from build123d import *

# Parameters (mm, degrees)
F0_W     = 105.55254668
F0_H     = 105.5525541306
F1_DEPTH = 99.314
F3_DEPTH = 104.14
F4_W     = 27.6781544089
F4_H     = 48.5944971442
F5_DEPTH = 3.81
F6_R     = 12.9022285529
F7_DEPTH = 4.826


with BuildPart() as f1:
    # F0 (on Top) → F1 (new body)
    with BuildSketch(Plane.XY):
        with Locations((0.8764155209, -6.7373067141)):
            Rectangle(F0_W, F0_H)
    extrude(amount=F1_DEPTH)

    # F2 (on face) → F3 (join)
    with BuildSketch(Plane(origin=(-51.8998578191, 0, 0), x_dir=(0, -1, 0), z_dir=(-1, 0, 0))):
        Polygon((12.3477084562, 113.1768599153), (-46.0389703512, 99.314), (59.5135837793, 99.314), align=None)
    extrude(amount=-F3_DEPTH)

    # F4 (on face) → F5 (cut)
    with BuildSketch(Plane.YZ.offset(53.6526888609)):
        with Locations((-5.462795496, 24.2972485721)):
            Rectangle(F4_W, F4_H)
    extrude(amount=-F5_DEPTH, mode=Mode.SUBTRACT)

    # F6 (on face) → F7 (cut)
    with BuildSketch(Plane.YZ.offset(53.6526888609)):
        with Locations((-9.2169223353, 78.1042650342)):
            Circle(F6_R)
    extrude(amount=-F7_DEPTH, mode=Mode.SUBTRACT)


solid = f1.part
For this review, take the finished solid that the model builds, in its own axes (mm). A direction names the side the tool comes from. Round coordinates to 2 decimals unless told otherwise and drop trailing zeros. Write each loop counter-clockwise with the first axis right and the second up, starting at its lowest first coordinate (ties: lowest second). Pieces come first, ordered by that corner, then holes. Notation, with made-up numbers: (41.25, -30) - (60.25, -30) arc R13 ccw to (60.25, -15) - close; hole circle Ø6 at (53, 64). An arc over 180 degrees is marked (long way). Write item = value, one per line. Start each with the question number.
1. Consider section D-D on z = 102.5. State the section outline as (x, y) points.
2. For faces 4 (the face through (48.827, -9, 78)), 5 (the face through (49.843, -6, 25)), 6 (the face through (52.24, -6, 103)), list the 3-axis set-ups (+Z, -Z, +X, -X, +Y, -Y) from which the entire face can be reached by the end or side of a thin tool; tool diameter is ignored.
3. Wall thickness on L1, parallel to X at y = -8, z = 87; L2, parallel to Z at x = 26, y = 10.5; L3, parallel to Z at x = 48, y = 1: over which ranges is each line inside the solid? List them lowest first.
4. Consider section A-A on x = -31. State the section outline as (y, z) points, plus the area to 3 significant figures.
5. Consider section C-C on y = -46. State the section outline as (x, z) points, plus the area to 3 significant figures.
6. For pin 1 Ø14 at (y, z) = (-7, 30.5) entering from +X; pin 2 Ø15 at (y, z) = (-29, 107.5) entering from +X; pin 3 Ø4 at (x, y) = (52.5, -4.5) entering from -Z, all flat-tipped, find the tip position at first contact; note any pin that passes through.
7. Consider section B-B on y = -17.5. State the section outline as (x, z) points, plus the area to 3 significant figures.
8. Draft analysis for pull direction Z (two halves, no side actions). For faces 1 (the face through (52, 8.376, 24)), 2 (the face through (51.27, 3.09, 81.98)), 3 (the face through (0, -6, 0)), state which applies: released by +Z, released by -Z, zero draft, split by the parting line, or undercut.
Evaluation:
q1.outline = (-51.9, -48.67) - (52.24, -48.67) - (52.24, 32.62) - (-51.9, 32.62) - close
q2.face_4 = +X
q2.face_5 = -Z, +X
q2.face_6 = +Z, +X, +Y, -Y
q3.L1 = -51.9 to 48.83
q3.L2 = 0 to 107.75
q3.L3 = 0 to 110.01
q4.outline = (-59.51, 0) - (46.04, 0) - (46.04, 99.31) - (-12.35, 113.18) - (-59.51, 99.31) - close
q4.area = 11,200 mm2
q5.outline = (-51.9, 0) - (53.65, 0) - (53.65, 99.31) - (52.24, 99.31) - (52.24, 103.29) - (-51.9, 103.29) - close
q5.area = 10,900 mm2
q6.pin_1 = 49.84
q6.pin_2 = 52.24
q6.pin_3 = 48.59
q7.outline = (-51.9, 0) - (49.84, 0) - (49.84, 48.59) - (53.65, 48.59) - (53.65, 68.21) - (48.83, 68.21) - (48.83, 88) - (53.65, 88) - (53.65, 99.31) - (52.24, 99.31) - (52.24, 111.66) - (-51.9, 111.66) - close
q7.area = 11,500 mm2
q8.face_1 = zero draft
q8.face_2 = undercut
q8.face_3 = released by -Z
